Geometry: final body of the model. Coordinates: model frame, mm. Face numbers are marked on the shaded views. A direction names the side the tool comes from. Give positions to 0.01 mm unless a question says otherwise; leave off trailing zeros. Order: outer loops, then holes, each group sorted by start corner. A loop starts at its lowest first (then second) coordinate and runs counter-clockwise, first axis right, second up. Notation, with made-up numbers: (-9, 78.5) - (1, 78.5) arc R17 cw to (1, 98.5) - close; hole circle Ø8 at (-27.5, -21). An arc over 180 degrees is marked (long way). Use one line per item in the form item = value.
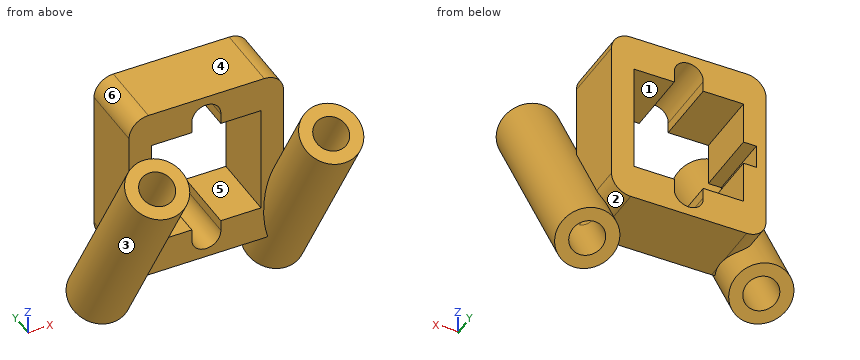
from build123d import *

# Parameters (mm, degrees)
F1_DEPTH      = 10.5
F4_R          = 4.625
F4_R_2        = 2.625
F5_DEPTH      = 20
F5_DEPTH_BACK = 15
F6_DEPTH      = 19.1738930562
F6_DEPTH_BACK = 25


with BuildPart() as f1:
    # F0 (on Front) → F1 (new body)
    with BuildSketch(Plane.XZ):
        with BuildLine():
            ThreePointArc((12, 10.924703002), (11.1213203436, 13.0460233455), (9, 13.924703002))
            Line((9, 13.924703002), (-9, 13.924703002))
            ThreePointArc((-9, 13.924703002), (-11.1213203436, 13.0460233455), (-12, 10.924703002))
            Line((-12, 10.924703002), (-12, -10.924703002))
            ThreePointArc((-12, -10.924703002), (-11.1213203436, -13.0460233455), (-9, -13.924703002))
            Line((-9, -13.924703002), (9, -13.924703002))
            ThreePointArc((9, -13.924703002), (11.1213203436, -13.0460233455), (12, -10.924703002))
            Line((12, -10.924703002), (12, 10.924703002))
        make_face()
        with BuildLine():
            Line((8.5, 8.5), (8.5, -8.5))
            Line((8.5, -8.5), (2.25, -8.5))
            Line((2.25, -8.5), (2.25, -10.1598765432))
            ThreePointArc((2.25, -10.1598765432), (0, -12.55), (-2.25, -10.1598765432))
            Line((-2.25, -10.1598765432), (-2.25, -8.5))
            Line((-2.25, -8.5), (-8.5, -8.5))
            Line((-8.5, -8.5), (-8.5, -1.85))
            Line((-8.5, -1.85), (-10.5, -1.85))
            Line((-10.5, -1.85), (-10.5, 1.85))
            Line((-10.5, 1.85), (-8.5, 1.85))
            Line((-8.5, 1.85), (-8.5, 8.5))
            Line((-8.5, 8.5), (-2.25, 8.5))
            Line((-2.25, 8.5), (-2.25, 10.1598765432))
            ThreePointArc((-2.25, 10.1598765432), (0, 12.55), (2.25, 10.1598765432))
            Line((2.25, 10.1598765432), (2.25, 8.5))
            Line((2.25, 8.5), (8.5, 8.5))
        make_face(mode=Mode.SUBTRACT)
    extrude(amount=F1_DEPTH)

    # F4 (on face) → F5 (join, two sides)
    with BuildSketch(Plane(origin=(0, 0, 0), x_dir=(1, 0, 0), z_dir=(0, 0.5, -0.8660254038))) as f5_sk:
        with Locations((13.525, 13.6721374395)):
            Circle(F4_R)
        with Locations((13.525, 13.6721374395)):
            Circle(F4_R_2, mode=Mode.SUBTRACT)
        with Locations((-13.525, 13.6721374395)):
            Circle(F4_R)
        with Locations((-13.525, 13.6721374395)):
            Circle(F4_R_2, mode=Mode.SUBTRACT)
    extrude(amount=-F5_DEPTH)
    extrude(f5_sk.sketch, amount=F5_DEPTH_BACK)

    # F4 (on face) → F6 (cut, two sides)
    with BuildSketch(Plane(origin=(0, 0, 0), x_dir=(1, 0, 0), z_dir=(0, 0.5, -0.8660254038))) as f6_sk:
        with Locations((-13.525, 13.6721374395)):
            Circle(F4_R_2)
        with Locations((13.525, 13.6721374395)):
            Circle(F4_R_2)
    extrude(amount=F6_DEPTH, mode=Mode.SUBTRACT)
    extrude(f6_sk.sketch, amount=-F6_DEPTH_BACK, mode=Mode.SUBTRACT)


solid = f1.part
(1) Pull-direction query (X, two-part tool) for the marked faces 4, 5 and 6; classes: released by +X, released by -X, zero draft, split by the parting line, or undercut.
Computed values:
face_4 = zero draft
face_5 = undercut
face_6 = released by -X
(2) Cut plane A-A on x = -7. Output: boundary loops of the cut face in (y, z), plus the area to 3 significant figures.
Computed values:
outline = (-10.5, -13.92) - (0, -13.92) - (0, -8.5) - (-10.5, -8.5) - close; (-10.5, 8.5) - (0, 8.5) - (0, 13.92) - (-10.5, 13.92) - close
area = 114 mm²
(3) Ray query, line 1 along Z through (x, y) = (5.5, -7.25); line 2 along X through (y, z) = (-5.5, -17); line 3 along Z through (x, y) = (0, -10). Return the intervals inside material, ascending.
Computed values:
line_1 = -13.92 to -8.5, 8.5 to 13.92
line_2 = -18.13 to -16.12, -10.93 to -8.92, 8.92 to 10.93, 16.12 to 18.13
line_3 = -13.92 to -12.55, 12.55 to 13.92
(4) Contact query for flat-ended pins moving along their axis: pin 1 Ø7.5 at (y, z) = (-3.5, 7) entering from +X; pin 2 Ø12 at (x, z) = (0, -12.5) entering from +Y; pin 3 Ø3 at (y, z) = (-6.5, 1.5) entering from -X; pin 4 Ø1.9 at (x, y) = (4, -3.5) entering from -Z. Output: stop coordinate, or through.
Computed values:
pin_1 = 12
pin_2 = 0
pin_3 = -12
pin_4 = -13.92
(5) Cut plane B-B on x = 0. Output: boundary loops of the cut face in (y, z).
Computed values:
outline = (-10.5, -13.92) - (0, -13.92) - (0, -12.55) - (-10.5, -12.55) - close; (-10.5, 12.55) - (0, 12.55) - (0, 13.92) - (-10.5, 13.92) - close
(6) Reachability of the marked faces 1, 2 and 3 from +Z, -Z, +X, -X, +Y, -Y: full face, straight path, thin tool, end or side. Return the list, or none.
Computed values:
face_1 = +Y, -Y
face_2 = +Y
face_3 = none
(7) Cut plane C-C on z = 9.5. Give the number of separate pieces and of enclosed holes in the cut face, plus the area to 3 significant figures.
Computed values:
separate_pieces = 4
enclosed_holes = 0
area = 277 mm²
